Autodesk Inventor part; units mm, degrees
ref_plane "YZ Plane" through (0, 0, 0) normal (1, 0, 0) x (0, 1, 0)
ref_plane "XZ Plane" through (0, 0, 0) normal (0, 1, 0) x (-1, 0, 0)
ref_plane "XY Plane" through (0, 0, 0) normal (0, 0, 1) x (1, 0, 0)
sketch "Sketch1" plane through (0, 0, 0) normal (0, 1, 0) x (-1, 0, 0)
  line L0 (-17.6137, 17.7414) -> (-15.5618, 16.2506)
  line L1 (-23.5374, 22.0452) -> (-13.679, 22.0452) construction
  line L2 (-22.316, 11.2693) -> (-20.2641, 9.7784)
  line L3 (-22.316, -11.2693) -> (-20.2641, -9.7784)
  line L4 (-17.6137, -17.7414) -> (-15.5618, -16.2506)
  line L5 (24.6779, 4) -> (22.1416, 4)
  line L6 (24.6779, -4) -> (22.1416, -4)
  line L7 (-20.2641, -9.7784) -> (-19.2354, -9.0311)
  line L8 (-15.5618, -16.2506) -> (-14.5332, -15.5032)
  line L9 (-20.2641, 9.7784) -> (-19.2354, 9.0311)
  line L10 (-15.5618, 16.2506) -> (-14.5332, 15.5032)
  line L11 (22.1416, 4) -> (20.8701, 4)
  line L12 (22.1416, -4) -> (20.8701, -4)
  arc A0 (-17.6137, -17.7414) -> (24.6779, -4) centre (0, 0) ccw
  arc A1 (24.6779, 4) -> (-17.6137, 17.7414) centre (0, 0) ccw
  arc A2 (-22.316, 11.2693) -> (-22.316, -11.2693) centre (0, 0) ccw
  line L13 (20.8701, 4) -> (15.8701, 4)
  line L14 (15.8701, 4) -> (15.8701, -4)
  line L15 (15.8701, -4) -> (20.8701, -4)
  line L16 (-14.5332, 15.5032) -> (-10.4881, 12.5643)
  line L17 (-10.4881, 12.5643) -> (-15.1903, 6.0922)
  line L18 (-15.1903, 6.0922) -> (-19.2354, 9.0311)
  line L19 (-19.2354, -9.0311) -> (-15.1903, -6.0922)
  line L20 (-15.1903, -6.0922) -> (-10.4881, -12.5643)
  line L21 (-10.4881, -12.5643) -> (-14.5332, -15.5032)
  circle A3 centre (-22.5, 0) radius 1.5
  circle A4 centre (0, 22.5) radius 1.5
  circle A5 centre (18.2029, 13.2252) radius 1.5
  circle A6 centre (18.2029, -13.2252) radius 1.5
  circle A7 centre (0, -22.5) radius 1.5
  circle A8 centre (0, 0) radius 4
  line L22 (0, 0) -> (8, 0)
  line L23 (8, 0) -> (8, 7.5)
  line L24 (8, 0) -> (8, -7.5)
  circle A9 centre (8, -7.5) radius 2.5
  circle A10 centre (8, 7.5) radius 2.5
  point P0 (-28.2397, -15.5731)
  point P1 (-23.5374, -22.0452)
  point P2 (32, -4)
  dimension "d1" = 36
  dimension "d3" = 5
  dimension "d4" = 5
  dimension "d6" = 3
  dimension "d7" = 3
  dimension "d8" = 3
  dimension "d9" = 3
  dimension "d10" = 3
  dimension "d13" = 8
  dimension "d14" = 8
  dimension "d15" = 7.5
  dimension "d16" = 7.5
  dimension "d17" = 5
  dimension "d18" = 5
extrude "Extrusion2" add sketch "Sketch1" along normal blind 3
properties part number "actuatorMountingPlate"
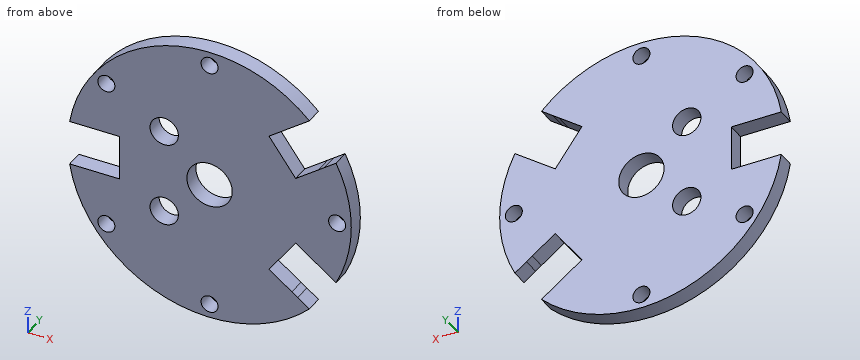
The listing builds one solid part. Answer for the finished solid, in the listing's coordinates (mm). Give positions to 0.01 mm unless a question says otherwise; leave off trailing zeros. Order: outer loops, then holes, each group sorted by start corner. A loop starts at its lowest first (then second) coordinate and runs counter-clockwise, first axis right, second up. Notation, with made-up numbers: (58.5, 73) -> (101.5, 73) arc R25 cw to (101.5, 105) -> close; hole circle Ø8 at (46.5, 71). An arc over 180 degrees is marked (long way). Put each result on its own line as item: value.
Item 1: Straight lines are drawn through the part: line 1 (Z direction, x = 0, y = 2.05); line 2 (X direction, y = 2.4, z = 8); line 3 (Z direction, x = 1, y = 0.75). For each, find the intervals that lie inside material, in ascending order.
Established:
line 1: z = -25 to -24, -21 to -4, 4 to 21, 24 to 25
line 2: x = -23.69 to -10.45, -5.55 to 13.8, 17.82 to 23.69
line 3: z = -24.98 to -23.62, -21.38 to -3.87, 3.87 to 21.38, 23.62 to 24.98
Item 2: A cutting plane is placed at B-B on x = 3. Give the vertices of the cut face in (y, z), plus the area to 3 significant figures.
Established:
outline: (0, -24.82) -> (3, -24.82) -> (3, -2.65) -> (0, -2.65) -> close; (0, 2.65) -> (3, 2.65) -> (3, 24.82) -> (0, 24.82) -> close
area: 133 mm^2
Item 3: A cutting plane is placed at D-D on y = 2.05. Count the separate pieces of the cut face and the enclosed holes in it, plus the area to 3 significant figures.
Established:
separate pieces: 1
enclosed holes: 8
area: 1,620 mm^2
Item 4: A cutting plane is placed at A-A on z = 0. Give the vertices of the cut face in (x, y).
Established:
outline: (-15.87, 0) -> (-4, 0) -> (-4, 3) -> (-15.87, 3) -> close; (4, 0) -> (21, 0) -> (21, 3) -> (4, 3) -> close; (24, 0) -> (25, 0) -> (25, 3) -> (24, 3) -> close
Item 5: Given P1, Ø1.5, axis at x = -21.5, y = 1, coming from the +Z side; P2, Ø1.5, axis at x = 9, y = 0.5, coming from the +Z side; P3, Ø1.5, axis at x = -22, y = 2, coming from the -Z side, each flat-ended and moving along its own axis, determine where each tip first touches the part or whether it passes through.
Established:
P1: stops at z = 13.94
P2: stops at z = 23.6
P3: stops at z = -13.17
Item 6: A cutting plane is placed at C-C on z = 22.5. Give the vertices of the cut face in (x, y).
Established:
outline: (-10.9, 0) -> (-1.5, 0) -> (-1.5, 3) -> (-10.9, 3) -> close; (1.5, 0) -> (10.9, 0) -> (10.9, 3) -> (1.5, 3) -> close
